Autodesk Inventor part; units mm, degrees
ref_plane "YZ Plane" through (0, 0, 0) normal (1, 0, 0) x (0, 1, 0)
ref_plane "XZ Plane" through (0, 0, 0) normal (0, 1, 0) x (-1, 0, 0)
ref_plane "XY Plane" through (0, 0, 0) normal (0, 0, 1) x (1, 0, 0)
sketch "Sketch1" plane through (0, 0, 0) normal (0, 0, 1) x (1, 0, 0)
  circle A0 centre (0, 0) radius 13.25
  circle A1 centre (0, 0) radius 4.5
  dimension "d0" = 26.5
  dimension "d1" = 9
extrude "Extrusion1" add sketch "Sketch1" along normal blind 5
sketch "Sketch2" plane through (0, 0, 5) normal (0, 0, 1) x (1, 0, 0)
  circle A0 centre (0, 10) radius 1.5
  circle A1 centre (0, -10) radius 1.5
  circle A2 centre (0, 0) radius 10 construction
  dimension "d4" = 3
  dimension "d5" = 3
  dimension "d6" = 20
extrude "Extrusion2" cut sketch "Sketch2" against normal through all
sketch "Sketch3" plane through (0, 0, 5) normal (0, 0, 1) x (1, 0, 0)
  circle A0 centre (0, 10) radius 1.5
  circle A1 centre (0, -10) radius 1.5
  circle A2 centre (0, 10) radius 3.5
  circle A3 centre (0, -10) radius 3.5
  point P0 (0, 0)
  dimension "d9" = 7
  dimension "d10" = 7
extrude "Extrusion3" cut sketch "Sketch3" against normal blind 3
properties part number "AA028" material "ABS Plastic"
Design review of the part built by this model. Coordinates are the model's own, in mm. A direction names the side the tool comes from. Give positions to 0.01 mm unless a question says otherwise; leave off trailing zeros. Write each loop counter-clockwise with the first axis right and the second up, starting at its lowest first coordinate (ties: lowest second). Pieces come first, ordered by that corner, then holes.
(1) Clearance check with flat-ended pins moving along their axes: pin 1 Ø3.5 at (x, y) = (1, -9.5) entering from +Z; pin 2 Ø1.5 at (y, z) = (-9.5, 4) entering from +X; pin 3 Ø2.5 at (x, y) = (0, 10) entering from +Z; pin 4 Ø1 at (x, z) = (-2, 4) entering from +Y. State where each tip first meets the part, or that it passes through.
Checked values:
pin 1: stops at z = 2
pin 2: stops at x = 9.95
pin 3: passes through
pin 4: stops at y = 13.16
(2) Mouldability with a two-part tool opening along Y and no side actions: class faces 3 (the face through (6, 0, 0)), 4 (the face through (-0.325, 8.536, 1.014)), 5 (the face through (7.123, -11.172, 2.465)) as +Y half, -Y half, draft (parallel to the pull), parting line (faces both ways), or undercut.
Checked values:
face 3: draft
face 4: undercut
face 5: parting line
(3) Tool access review of faces 1 (the face through (0, 8, 2)), 2 (the face through (6, 0, 5)): name each direction out of +Z, -Z, +X, -X, +Y, -Y from which nothing blocks a thin tool from reaching the whole face with its end or side.
Checked values:
face 1: +Z
face 2: +Z, +X, -X, +Y, -Y
(4) Wall thickness on line 1 along Y through (x, z) = (0, 0.75); line 2 along X through (y, z) = (0.25, 3.25); line 3 along Y through (x, z) = (0, 4.1): over which ranges is each line inside the solid? List them lowest first.
Checked values:
line 1: y = -13.25 to -11.5, -8.5 to -4.5, 4.5 to 8.5, 11.5 to 13.25
line 2: x = -13.25 to -4.49, 4.49 to 13.25
line 3: y = -6.5 to -4.5, 4.5 to 6.5
(5) Add section C-C (z = 1.45). Give the boundary of the cut face in (x, y).
Checked values:
outline: circle Ø26.5 at (0, 0); hole circle Ø9 at (0, 0); hole circle Ø3 at (0, -10); hole circle Ø3 at (0, 10)
(6) Add section D-D (x = 3). Give the boundary of the cut face in (y, z), and give its area (3 significant figures).
Checked values:
outline: (-12.91, 0) - (-3.35, 0) - (-3.35, 5) - (-8.2, 5) - (-8.2, 2) - (-11.8, 2) - (-11.8, 5) - (-12.91, 5) - close; (3.35, 0) - (12.91, 0) - (12.91, 5) - (11.8, 5) - (11.8, 2) - (8.2, 2) - (8.2, 5) - (3.35, 5) - close
area: 73.9 mm2
(7) Add section B-B (y = 0). Give the boundary of the cut face in (x, z), and give its area (3 significant figures).
Checked values:
outline: (-13.25, 0) - (-4.5, 0) - (-4.5, 5) - (-13.25, 5) - close; (4.5, 0) - (13.25, 0) - (13.25, 5) - (4.5, 5) - close
area: 87.5 mm2
(8) Add section A-A (x = 0). Give the boundary of the cut face in (y, z), and give its area (3 significant figures).
Checked values:
outline: (-13.25, 0) - (-11.5, 0) - (-11.5, 2) - (-13.25, 2) - close; (-8.5, 0) - (-4.5, 0) - (-4.5, 5) - (-6.5, 5) - (-6.5, 2) - (-8.5, 2) - close; (4.5, 0) - (8.5, 0) - (8.5, 2) - (6.5, 2) - (6.5, 5) - (4.5, 5) - close; (11.5, 0) - (13.25, 0) - (13.25, 2) - (11.5, 2) - close
area: 35.0 mm2
